CAD build for the part. Positions are in the model's coordinates, mm. Coordinates: 2 decimals unless noted, no trailing zeros. Loops run counter-clockwise (first coordinate to the right, second up) from the corner with the lowest first, then second, coordinate; pieces in that order, holes last.
1) Wall check: line 1 along Z through (x, y) = (-7, -0.8); line 2 along Z through (x, y) = (-58.5, 1.8); line 3 along Z through (x, y) = (-58.5, -1.4). Give the ranges that are in metal, low to high.
2) Saw through at B-B, the plane z = 43.5. Write the cut outline in (x, y), and give its area (3 significant figures).
3) Saw through at A-A, the plane x = -17.5. Write the cut outline in (y, z).
4) Saw through at C-C, the plane y = -1.25. Give the number of separate pieces and of enclosed holes in the cut face, and give its area (3 significant figures).
5) Pin check, flat tips, straight feed: pin 1 Ø1 at (x, z) = (-28, -25) entering from +Y; pin 2 Ø1.5 at (y, z) = (-1.5, -34) entering from +X. Stop position of each tip, or through.
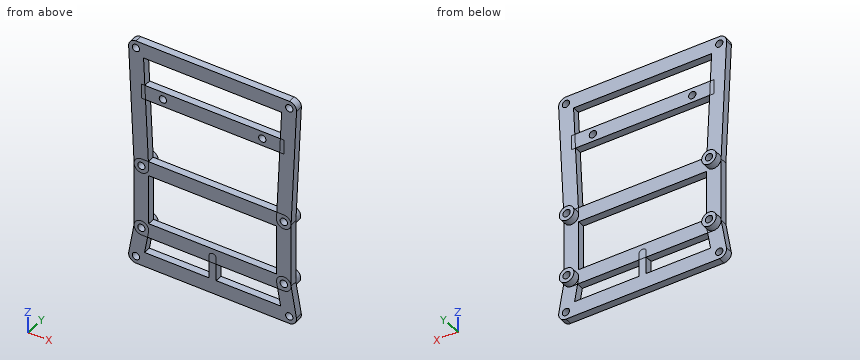
Autodesk Inventor part; units mm, degrees
ref_plane "YZ Plane" through (0, 0, 0) normal (1, 0, 0) x (0, 1, 0)
ref_plane "XZ Plane" through (0, 0, 0) normal (0, 1, 0) x (-1, 0, 0)
ref_plane "XY Plane" through (0, 0, 0) normal (0, 0, 1) x (1, 0, 0)
sketch "Sketch1" plane through (0, 0, 0) normal (0, 1, 0) x (-1, 0, 0)
  line L0 (0, 0) -> (58.5, 0)
  line L1 (58.5, 0) -> (58.5, -26.5)
  line L2 (58.5, -26.5) -> (0, -26.5)
  line L3 (0, -26.5) -> (0, 0)
  circle A0 centre (58.5, 0) radius 1.5
  circle A1 centre (58.5, -26.5) radius 1.5
  circle A2 centre (0, 0) radius 1.5
  circle A3 centre (0, -26.5) radius 1.5
  circle A4 centre (0, 0) radius 3
  circle A5 centre (0, -26.5) radius 3
  circle A6 centre (58.5, 0) radius 3
  circle A7 centre (58.5, -26.5) radius 3
  dimension "d0" = 58.5
  dimension "d1" = 26.5
  dimension "d2" = 3
  dimension "d3" = 3
  dimension "d4" = 3
  dimension "d5" = 3
  dimension "d6" = 6
  dimension "d7" = 6
  dimension "d8" = 6
  dimension "d9" = 6
extrude "Extrusion1" add sketch "Sketch1" along normal blind 3 contours A2 L3 A4 L0 | L0 A4 L3 A2 | A6 L1 A0 L0 | L0 A0 L1 A6 | A5 L2 A3 L3 | L3 A3 L2 A5 | A7 L2 A1 L1 | L1 A1 L2 A7
sketch "Sketch2" plane through (0, 0, 0) normal (0, -1, 0) x (1, 0, 0)
  circle A0 centre (0, 0) radius 1.5
  circle A1 centre (0, -26.5) radius 1.5
  circle A2 centre (0, -26.5) radius 1.5
  circle A3 centre (-58.5, -26.5) radius 1.5
  circle A4 centre (-58.5, -26.5) radius 1.5
  circle A5 centre (-58.5, 0) radius 1.5
  circle A6 centre (-58.5, 0) radius 1.5
  line L0 (-58.5, 0) -> (0, 0) construction
  line L1 (-58.5, -3) -> (0, -3)
  line L2 (0, 3) -> (-58.5, 3)
  arc A7 (-58.5, 3) -> (-58.5, -3) centre (-58.5, 0) ccw
  arc A8 (0, -3) -> (0, 3) centre (0, 0) ccw
  line L3 (0, 0) -> (0, -26.5) construction
  line L4 (-3, 0) -> (-3, -26.5)
  line L5 (3, -26.5) -> (3, 0)
  arc A9 (3, 0) -> (-3, 0) centre (0, 0) ccw
  arc A10 (-3, -26.5) -> (3, -26.5) centre (0, -26.5) ccw
  line L6 (0, -26.5) -> (-58.5, -26.5) construction
  line L7 (0, -29.5) -> (-58.5, -29.5)
  line L8 (-58.5, -23.5) -> (0, -23.5)
  arc A11 (0, -29.5) -> (0, -23.5) centre (0, -26.5) ccw
  arc A12 (-58.5, -23.5) -> (-58.5, -29.5) centre (-58.5, -26.5) ccw
  line L9 (-58.5, -26.5) -> (-58.5, 0) construction
  line L10 (-55.5, -26.5) -> (-55.5, 0)
  line L11 (-61.5, 0) -> (-61.5, -26.5)
  arc A13 (-61.5, -26.5) -> (-55.5, -26.5) centre (-58.5, -26.5) ccw
  arc A14 (-55.5, 0) -> (-61.5, 0) centre (-58.5, 0) ccw
  point P0 (-29.25, 0)
  point P1 (0, -13.25)
  point P2 (-29.25, -26.5)
  point P3 (-58.5, -13.25)
  point P4 (-3, -3)
  point P5 (-3, -23.5)
  point P6 (-55.5, -23.5)
  point P7 (-55.5, -3)
extrude "Extrusion2" add sketch "Sketch2" along normal blind 3 contours A7 A14 L10 L1 | L1 L10 L8 A12 L11 A7 | L10 A14 L2 A9 L4 L1 | L4 A9 A8 L1 | L1 A8 L5 A11 L8 L4 | L10 A13 A12 L8 | L8 L4 A10 L7 A13 L10 | L8 A11 A10 L4
sketch "Sketch3" plane through (0, -3, 0) normal (0, -1, 0) x (1, 0, 0)
  line L0 (-58.5, -29.5) -> (0, -29.5)
  line L1 (-29.25, -29.5) -> (-29.25, -39.5)
  line L2 (-60.75, -39.5) -> (2.25, -39.5)
  circle A0 centre (-60.75, -39.5) radius 1.5
  circle A1 centre (2.25, -39.5) radius 1.5
  circle A2 centre (-58.5, -26.5) radius 1.5
  line L3 (-60.75, -39.5) -> (-58.5, -26.5) construction
  line L4 (-57.7939, -40.0116) -> (-55.5439, -27.0116)
  line L5 (-61.4561, -25.9884) -> (-63.7061, -38.9884)
  arc A3 (-63.7061, -38.9884) -> (-57.7939, -40.0116) centre (-60.75, -39.5) ccw
  arc A4 (-55.5439, -27.0116) -> (-61.4561, -25.9884) centre (-58.5, -26.5) ccw
  circle A5 centre (0, -26.5) radius 1.5
  line L6 (2.25, -39.5) -> (0, -26.5) construction
  line L7 (5.2061, -38.9884) -> (2.9561, -25.9884)
  line L8 (-2.9561, -27.0116) -> (-0.7061, -40.0116)
  arc A6 (-0.7061, -40.0116) -> (5.2061, -38.9884) centre (2.25, -39.5) ccw
  arc A7 (2.9561, -25.9884) -> (-2.9561, -27.0116) centre (0, -26.5) ccw
  line L9 (-60.75, -39.5) -> (2.25, -39.5) construction
  line L10 (-60.75, -36.5) -> (2.25, -36.5)
  line L11 (2.25, -42.5) -> (-60.75, -42.5)
  arc A8 (-60.75, -36.5) -> (-60.75, -42.5) centre (-60.75, -39.5) ccw
  arc A9 (2.25, -42.5) -> (2.25, -36.5) centre (2.25, -39.5) ccw
  line L12 (-29.25, -39.5) -> (-29.25, -27.0116) construction
  line L13 (-27.75, -39.5) -> (-27.75, -27.0116)
  line L14 (-30.75, -27.0116) -> (-30.75, -39.5)
  arc A10 (-30.75, -39.5) -> (-27.75, -39.5) centre (-29.25, -39.5) ccw
  arc A11 (-27.75, -27.0116) -> (-30.75, -27.0116) centre (-29.25, -27.0116) ccw
  point P0 (0, 0)
  point P1 (-59.625, -33)
  point P2 (1.125, -33)
  point P3 (-29.25, -33.2558)
  point P4 (-57.1862, -36.5)
  point P5 (-1.3138, -36.5)
  point P6 (-27.75, -36.5)
  point P7 (-30.75, -36.5)
  dimension "d14" = 10
  dimension "d15" = 63
  dimension "d16" = 3
  dimension "d17" = 3
  dimension "d18" = 6
  dimension "d19" = 6
  dimension "d20" = 3
extrude "Extrusion3" add sketch "Sketch3" against normal blind 3 contours L4 L10 A8 L5 A4 | L14 A11 L13 L0 | L0 L1 L10 L14 | L10 L14 L2 L4 | L4 A3 A8 L10 | L0 L13 L10 L1 | L10 L1 L2 L14 | L2 A10 L8 A6 L11 A3 L4 | L10 L13 L2 L1 | L2 A10 | L8 A7 L7 A9 L10 | L10 L8 L2 L13 | L10 A9 A6 L8
sketch "Sketch4" plane through (0, 0, 0) normal (0, 1, 0) x (1, 0, 0)
  circle A0 centre (2.25, 39.5) radius 1.5
  line L0 (2.25, 39.5) -> (2.25, -49.5)
  line L1 (2.25, -49.5) -> (-60.75, -49.5)
  circle A1 centre (2.25, -49.5) radius 1.5
  circle A2 centre (-60.75, -49.5) radius 1.5
  circle A3 centre (-58.5, 0) radius 1.5
  line L2 (-60.75, -49.5) -> (-58.5, 0) construction
  line L3 (-57.7531, -49.6362) -> (-55.5031, -0.1362)
  line L4 (-61.4969, 0.1362) -> (-63.7469, -49.3638)
  arc A4 (-63.7469, -49.3638) -> (-57.7531, -49.6362) centre (-60.75, -49.5) ccw
  arc A5 (-55.5031, -0.1362) -> (-61.4969, 0.1362) centre (-58.5, 0) ccw
  line L5 (2.25, -49.5) -> (0, 0) construction
  line L6 (5.2469, -49.3638) -> (2.9969, 0.1362)
  line L7 (-2.9969, -0.1362) -> (-0.7469, -49.6362)
  arc A6 (-0.7469, -49.6362) -> (5.2469, -49.3638) centre (2.25, -49.5) ccw
  arc A7 (2.9969, 0.1362) -> (-2.9969, -0.1362) centre (0, 0) ccw
  line L8 (2.25, -49.5) -> (-60.75, -49.5) construction
  line L9 (2.25, -46.5) -> (-60.75, -46.5)
  line L10 (-60.75, -52.5) -> (2.25, -52.5)
  arc A8 (2.25, -52.5) -> (2.25, -46.5) centre (2.25, -49.5) ccw
  arc A9 (-60.75, -46.5) -> (-60.75, -52.5) centre (-60.75, -49.5) ccw
  circle A10 centre (0, 0) radius 1.5
  circle A11 centre (-58.5, 0) radius 1.5
  point P0 (-59.625, -24.75)
  point P1 (1.125, -24.75)
  point P2 (-29.25, -49.5)
  point P3 (-0.8895, -46.5)
  point P4 (-57.6105, -46.5)
  point P5 (2.25, -52.5)
  dimension "d23" = 89
  dimension "d24" = 63
  dimension "d25" = 3
  dimension "d26" = 3
  dimension "d27" = 6
  dimension "d28" = 6
extrude "Extrusion4" add sketch "Sketch4" against normal blind 3 contours A7 L6 A8 L0 | L0 L9 L7 A7 | A8 A6 L7 L1 A1 L0 | L0 A1 L1 L7 L9 | L7 L1 L3 L9 | L7 A6 L10 A4 L3 L1 | L9 A9 L4 A5 L3 | L3 A4 A9 L9
sketch "Sketch5" plane through (0, 0, 0) normal (0, 1, 0) x (1, 0, 0)
  circle A0 centre (-58.5, 0) radius 1.5
  line L0 (-58.5, 0) -> (0, 0)
  line L1 (0, 0) -> (0, -35)
  line L2 (0, -35) -> (-58.5, -35)
  line L3 (-58.5, -35) -> (-58.5, 0)
  line L4 (0, -35) -> (-58.5, -35)
  line L5 (-58.5, -35) -> (-58.5, -29)
  line L6 (-58.5, -29) -> (0, -29)
  line L7 (0, -29) -> (0, -35)
  line L8 (-29.25, -29) -> (-29.25, -35)
  line L9 (-49.672, -32) -> (-8.828, -32)
  circle A1 centre (-49.672, -32) radius 1.5
  circle A2 centre (-8.828, -32) radius 1.5
  point P0 (-29.25, -32)
  point P1 (0, -29)
  dimension "d31" = 35
  dimension "d32" = 6
  dimension "d33" = 40.844
  dimension "d34" = 3
  dimension "d35" = 3
extrude "Extrusion5" add sketch "Sketch5" against normal blind 3 contours L6 L8 L2 L3 | L1 L2 L8 L6
properties part number "bigbucksupport"
Data:
1. line 1: z = -42.5 to -36.5, -29.5 to -23.5, -3 to 3, 29 to 35, 46.5 to 52.5
1. line 2: z = -29.5 to -28, -25 to -23.5, -3 to -1.5, 1.5 to 3
1. line 3: z = -42.5 to -28, -25 to -1.5, 1.5 to 52.5
2. outline: (-63.48, -3) - (-57.47, -3) - (-57.47, 0) - (-63.48, 0) - close; (-1.03, -3) - (4.98, -3) - (4.98, 0) - (-1.03, 0) - close
2. area: 36.0 mm2
3. outline: (-3, -42.5) - (0, -42.5) - (0, -36.5) - (-3, -36.5) - close; (-3, -29.5) - (0, -29.5) - (0, -23.5) - (-3, -23.5) - close; (-3, -3) - (0, -3) - (0, 3) - (-3, 3) - close; (-3, 29) - (0, 29) - (0, 35) - (-3, 35) - close; (-3, 46.5) - (0, 46.5) - (0, 52.5) - (-3, 52.5) - close
4. separate pieces: 1
4. enclosed holes: 15
4. area: 2,730 mm2
5. pin 1: stops at y = 0
5. pin 2: stops at x = 4.47
